```python
from build123d import *

# Parameters (mm, degrees)
F0_W     = 25.4
F0_H     = 25.4
F1_DEPTH = 12.7
F2_R     = 9.525
F3_DEPTH = 10.16
F4_R     = 8.255
F5_DEPTH = 2.541
F6_R     = 1.905
F7_DEPTH = 12.701
F8_R     = 2.205983
F9_DEPTH = 12.701


with BuildPart() as f1:
    # F0 (on Top) → F1 (new body)
    with BuildSketch(Plane.XY):
        with Locations((12.7, 12.7)):
            Rectangle(F0_W, F0_H)
    extrude(amount=F1_DEPTH)

    # F2 (on face) → F3 (cut)
    with BuildSketch(Plane.XY.offset(12.7)):
        with Locations((12.7, 12.7)):
            Circle(F2_R)
    extrude(amount=-F3_DEPTH, mode=Mode.SUBTRACT)

    # F4 (on face) → F5 (cut, through all)
    with BuildSketch(Plane.XY.offset(2.54)):
        with Locations((12.7, 12.7)):
            Circle(F4_R)
    extrude(amount=-F5_DEPTH, mode=Mode.SUBTRACT)

    # F6 (on face) → F7 (cut, through all)
    with BuildSketch(Plane.XY.offset(12.7)):
        with Locations((2.54899, 3.257044)):
            Circle(F6_R)
    extrude(amount=-F7_DEPTH, mode=Mode.SUBTRACT)

    # F8 (on face) → F9 (cut, through all)
    with BuildSketch(Plane.XY.offset(12.7)):
        with Locations((22.317057, 2.864695)):
            Circle(F8_R)
    extrude(amount=-F9_DEPTH, mode=Mode.SUBTRACT)


solid = f1.part
```
Can you work these out from the model? Positions are in its coordinate system, mm. A direction names the side the tool comes from. Give positions to 0.01 mm unless a question says otherwise; leave off trailing zeros. Order: outer loops, then holes, each group sorted by start corner. A loop starts at its lowest first (then second) coordinate and runs counter-clockwise, first axis right, second up. Notation, with made-up numbers: M 46,-25 L 87,-25 A24 ccw 87,-8 Z; hole C 43,-18.75 d6. An arc over 180 degrees is marked long. Write item = value, one per line. Start each with the question number.
Q1. Suppose I cut it at D-D (x = 2). Write out the boundary of the cut face in (y, z), plus the area to 3 significant figures.
Q2. I need wall thicknesses on probe 1 along Y at (x, z) = (12.7, 0.6) (3 decimals); probe 2 along X at (y, z) = (4.25, 10.5); probe 3 along X at (y, z) = (16.75, 4.5). Which ranges of each line are inside material? Lowest first, please. Write a range as [from, to].
Q3. Suppose I cut it at A-A (x = 12.7). Write out the boundary of the cut face in (y, z) (3 decimals), plus the area to 3 significant figures.
Q4. For faces 4 (the flat face through (10, 21, 2.54)), 5 (the flat face through (25.4, 13, 6)), which set-ups out of +Z, -Z, +X, -X, +Y, -Y let a thin tool reach every point of the face, with its end or its side?
Q5. Suppose I cut it at C-C (z = 7). Write out the boundary of the cut face in (x, y) (3 decimals), plus the area to 3 significant figures.
Q6. We'd pull the mould along Y, two halves only. Please class faces 1 (the flat face through (13, 25.4, 6)), 2 (the cylindrical face through (10.64, 3.4, 7.69)), 3 (the flat face through (0, 13, 6)): pulls with the +Y half, pulls with the -Y half, needs draft (parallel to the pull), parting line crosses it, or undercut.
Check result:
q1.outline = M 0,0 L 1.43,0 L 1.43,12.7 L 0,12.7 Z; M 5.08,0 L 25.4,0 L 25.4,12.7 L 5.08,12.7 Z
q1.area = 276 mm2
q2.probe_1 = [0, 4.445], [20.955, 25.4]
q2.probe_2 = [0, 0.92], [4.17, 8.3], [17.1, 20.6], [24.03, 25.4]
q2.probe_3 = [0, 4.08], [21.32, 25.4]
q3.outline = M 0,0 L 4.445,0 L 4.445,2.54 L 3.175,2.54 L 3.175,12.7 L 0,12.7 Z; M 20.955,0 L 25.4,0 L 25.4,12.7 L 22.225,12.7 L 22.225,2.54 L 20.955,2.54 Z
q3.area = 87.1 mm2
q4.face_4 = +Z
q4.face_5 = +Z, -Z, +X, +Y, -Y
q5.outline = M 0,0 L 25.4,0 L 25.4,25.4 L 0,25.4 Z; hole C 2.549,3.257 d3.81; hole C 12.7,12.7 d19.05; hole C 22.317,2.865 d4.412
q5.area = 333 mm2
q6.face_1 = pulls with the +Y half
q6.face_2 = undercut
q6.face_3 = needs draft
